```python
from build123d import *

# Parameters (mm, degrees)
BOSS_EXTRUDE2_DEPTH = 109.73
SKETCH2_R           = 2.5
CUT_EXTRUDE1_DEPTH  = 10


with BuildPart() as part:
    # Sketch1 → Boss-Extrude2 (new body)
    with BuildSketch(Plane.XY):
        Polygon((-10, 0.391567614), (-10, -3.576580006), (-10, -8.108432386), (10, -8.108432386), (10, 0.391567614), (6.5, 0.391567614), (6.5, -0.608432386), (8.5, -0.608432386), (8.5, -5.108432386), (-8.5, -5.108432386), (-8.5, -0.608432386), (-6.5, -0.608432386), (-6.5, 0.391567614), align=None)
    extrude(amount=BOSS_EXTRUDE2_DEPTH)

    # Sketch2 → Cut-Extrude1 (cut)
    with BuildSketch(Plane.XZ.offset(8.108432386)):
        with Locations((0, 30)):
            Circle(SKETCH2_R)
        with Locations((0, 80)):
            Circle(SKETCH2_R)
    extrude(amount=-CUT_EXTRUDE1_DEPTH, mode=Mode.SUBTRACT)


solid = part.part
```
CAD build for the part. Positions are in the model's coordinates, mm. A direction names the side the tool comes from. Coordinates: 2 decimals unless noted, no trailing zeros. Order: outer loops, then holes, each group sorted by start corner. A loop starts at its lowest first (then second) coordinate and runs counter-clockwise, first axis right, second up. Notation, with made-up numbers: M 42.5,87.25 L 89.5,87.25 A34 cw 89.5,126.25 Z; hole C 29.25,59.5 d2. An arc over 180 degrees is marked long. Write each question's results on one line, items separated by ' | '. Start each with the question number.
Q1. Cut at A-A (x = 0). List the corners of the cut face in (y, z).
Q2. Flat gauge pins, fed straight in: P1, Ø8.5, axis at x = -2.5, z = 78, coming from the +Y side; P2, Ø6, axis at x = 0, z = 30, coming from the +Y side. Where does each tip first touch, or does it go through?
Q3. Cut at B-B (z = 30). List the corners of the cut face in (x, y).
Q4. Cut at C-C (z = 90.5). List the corners of the cut face in (x, y).
Q5. Which spindle directions (+Z, -Z, +X, -X, +Y, -Y) get a long thin tool onto all of the face, cutting with end or side? Do faces 5 (the flat face through (-8, -0.608, 54)), 6 (the flat face through (-10, -4, 54)). Say none if no direction does.
Q6. Drill centre lines: probe 1 along Z at (x, y) = (0, -5.9); probe 2 along X at (y, z) = (0, 25.5); probe 3 along Y at (x, z) = (6.75, 102.5). Where is each one in solid material? Low to high. Write a range as from..to.
Q7. Pull direction Z, two halves, no side cores. Call faces 1 (the cylindrical face through (1.15, -6.63, 77.78)), 2 (the flat face through (0, -6, 0)), 3 (the flat face through (0, -6, 109.73)), 4 (the flat face through (7, -0.608, 54)): +Z half, -Z half, draft (parallel to the pull), parting line (faces both ways), or undercut.
Q8. Cut at D-D (x = 4.5). List the corners of the cut face in (y, z).
Found:
1) outline: M -8.11,0 L -5.11,0 L -5.11,27.5 L -8.11,27.5 Z; M -8.11,32.5 L -5.11,32.5 L -5.11,77.5 L -8.11,77.5 Z; M -8.11,82.5 L -5.11,82.5 L -5.11,109.73 L -8.11,109.73 Z
2) P1: y = 0.39 | P2: y = -5.11
3) outline: M -10,-8.11 L -2.5,-8.11 L -2.5,-5.11 L -8.5,-5.11 L -8.5,-0.61 L -6.5,-0.61 L -6.5,0.39 L -10,0.39 Z; M 2.5,-8.11 L 10,-8.11 L 10,0.39 L 6.5,0.39 L 6.5,-0.61 L 8.5,-0.61 L 8.5,-5.11 L 2.5,-5.11 Z
4) outline: M -10,-8.11 L 10,-8.11 L 10,0.39 L 6.5,0.39 L 6.5,-0.61 L 8.5,-0.61 L 8.5,-5.11 L -8.5,-5.11 L -8.5,-0.61 L -6.5,-0.61 L -6.5,0.39 L -10,0.39 Z
5) face 5: +Z, -Z | face 6: +Z, -Z, -X, +Y, -Y
6) probe 1: 0..27.5, 32.5..77.5, 82.5..109.73 | probe 2: -10..-6.5, 6.5..10 | probe 3: -8.11..-5.11, -0.61..0.39
7) face 1: undercut | face 2: -Z half | face 3: +Z half | face 4: draft
8) outline: M -8.11,0 L -5.11,0 L -5.11,109.73 L -8.11,109.73 Z
